Autodesk Inventor part; units mm, degrees
ref_plane "Work Plane1" through (29, 0, 0) normal (0, -1, 0) x (1, 0, 0)
ref_plane "YZ Plane" through (0, 0, 0) normal (1, 0, 0) x (0, 1, 0)
ref_plane "XZ Plane" through (0, 0, 0) normal (0, 1, 0) x (-1, 0, 0)
sketch "Sketch1" plane through (0, 0, 0) normal (0, 0, 1) x (1, 0, 0)
  line L0 (-1.3333, 0) -> (40, 0)
  line L1 (40, 0) -> (40, 3)
  line L2 (40, 3) -> (22, 3)
  line L3 (22, 3) -> (21.3865, 3)
  line L4 (21.3865, 3) -> (0, 3)
  line L5 (0, 3) -> (0, 5)
  line L6 (0, 5) -> (-6, 5)
  line L7 (-6, 5) -> (-6, 2.8868)
  line L8 (-6, 2.8868) -> (-3, 2.8868)
  line L9 (-3, 2.8868) -> (-1.3333, 0)
  line L10 (-15.2, 0) -> (49.2, 0)
  line L11 (0, -1) -> (0, 6)
  line L12 (22, 3) -> (0, 3) construction
  dimension "d1" = 18
  dimension "d2" = 0.6136
  dimension "d3" = 6
  dimension "d4" = 3
  dimension "d5" = 60
  dimension "d6" = 6
  dimension "d7" = 6
  dimension "d8" = 5.7735
  dimension "d9" = 10
  dimension "d26" = 40
revolve "Body" add sketch "Sketch1" angle 360 about axis through (-1.3333, 0, 0) along (1, 0, 0)
sketch "Sketch2" plane through (-6, 0, 0) normal (-1, 0, 0) x (0, 0, 1)
  circle A0 centre (0, 0) radius 2.8868
  line L0 (0, -7) -> (0, 7)
  line L1 (-7, 0) -> (7, 0)
  line L2 (2.8868, 0) -> (1.4434, -2.5)
  line L3 (1.4434, -2.5) -> (-1.4434, -2.5)
  line L4 (-1.4434, -2.5) -> (-2.8868, 0)
  line L5 (-2.8868, 0) -> (-1.4434, 2.5)
  line L6 (-1.4434, 2.5) -> (1.4434, 2.5)
  line L7 (1.4434, 2.5) -> (2.8868, 0)
extrude "Slot" add sketch "Sketch2" against normal up to next contours L7 A0 | A0 L2 | L6 L0 A0 | A0 L0 L3 | L0 L6 A0 | A0 L3 L0 | L4 A0 | A0 L5
fillet "Fillet1" radius 0.6 1 edges at (-6, -5, 0)
thread "Thread"
chamfer "Chamfer1" distance 0.6135 distance2 0.6135 1 edges at (40, -3, 0) measured on face at (40, -0.7485, 0.6631)
ref_plane "Work Plane1" through (29, 0, 0) normal (0, -1, 0) x (1, 0, 0)
fillet "Fillet2" radius 0.1 1 edges at (0, -3, 0)
equation "\"d1\" = GEL"
equation "\"d3\" = KOH"
equation "\"d4\" = INTI"
equation "\"d6\" = GD"
equation "\"d7\" = BDM"
equation "\"d8\" = 1.1547 * SW"
equation "\"d9\" = KOD"
equation "\"d26\" = NLG"
equation "\"d30\" = R"
equation "\"d17\" = RR"
equation "\"d13\" = GEL"
equation "\"d15\" = -0.5 * SPD + 0.5 * GD"
equation "\"d16\" = GUL"
equation "\"GD\" = NND"
equation "\"NLG\" = 40"
equation "\"GEL\" = 18"
equation "\"KOD\" = 10"
equation "\"KOH\" = NND"
equation "\"INTI\" = 3"
equation "\"GAL\" = 0.61345 * PTC"
equation "\"GUL\" = 0.61345 * PTC"
equation "\"BDM\" = NND"
equation "\"SW\" = 5"
equation "\"RR\" = 0.1 * NND"
equation "\"SPD\" = NND - 1.2269 * PTC"
equation "\"R\" = 0.1"
equation "\"PHH\" = 0.2"
equation "\"GD1\" = THREADDIA - 1.2269 * PTC"
equation "\"THREADDIA\" = 6"
equation "\"FAWI\" = 45deg"
equation "\"PTC\" = 1"
equation "\"KOH1\" = 5.4"
equation "\"NND\" = 6"
equation "\"TOA\" = 30deg"
equation "\"E0\" = 1.155 * SW"
properties part number "AS 1420 - 1973 - M6 x 40" material "Steel, Mild"
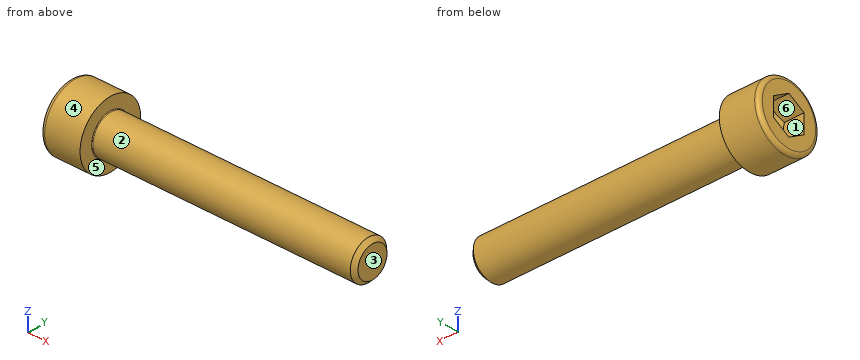
Read the model definition and answer for the solid it produces. Units are mm, in the model's axes. Face numbers are marked on the shaded views. A direction names the side the tool comes from. Coordinates: 2 decimals unless noted, no trailing zeros. Loops run counter-clockwise (first coordinate to the right, second up) from the corner with the lowest first, then second, coordinate; pieces in that order, holes last. Notation, with made-up numbers: (-16.75, -24) -> (32.25, -24) arc R17 cw to (32.25, -4) -> close; hole circle Ø11 at (82, 23). An arc over 180 degrees is marked (long way). Answer in a Markdown table with one row per item.
Item 1: Each of these flat-tipped pins is pushed along its axis until it touches: P1, Ø5, axis at x = 6, y = 0, coming from the +Z side; P2, Ø1, axis at x = 30, z = 3, coming from the -Y side; P3, Ø2, axis at x = 6, z = 1.5, coming from the -Y side. Where does it stop, or does it pass through?
Returned:
| item | result |
|---|---|
| P1 | stops at z = 3 |
| P2 | stops at y = -1.66 |
| P3 | stops at y = -2.96 |
Item 2: For a pull along Y with two mould halves and no side action, classify the marked faces 4, 5 and 6 as released by +Y, released by -Y, zero draft, split by the parting line, or undercut.
Returned:
| item | result |
|---|---|
| face 4 | split by the parting line |
| face 5 | zero draft |
| face 6 | undercut |
Item 3: For the marked faces 1, 2 and 3, determine the directions among +Z, -Z, +X, -X, +Y, -Y from which every point of the face is accessible in a straight line to the end or side of a thin tool.
Returned:
| item | result |
|---|---|
| face 1 | -X |
| face 2 | +X |
| face 3 | +Z, -Z, +X, +Y, -Y |
Item 4: A cutting plane is placed at A-A on x = 23.5. Determine the outline of the cut face in (y, z).
Returned:
| item | result |
|---|---|
| outline | circle Ø6 at (0, 0) |
Item 5: Straight lines are drawn through the part: line 1 along X through (y, z) = (2, 3.5); line 2 along Y through (x, z) = (-4, -0.5); line 3 along Z through (x, y) = (23.5, -2.25). For each, find the intervals that lie inside material, in ascending order. Write a range as [from, to].
Returned:
| item | result |
|---|---|
| line 1 | x = [-6, 0] |
| line 2 | y = [-4.97, -2.5], [2.5, 4.97] |
| line 3 | z = [-1.98, 1.98] |
